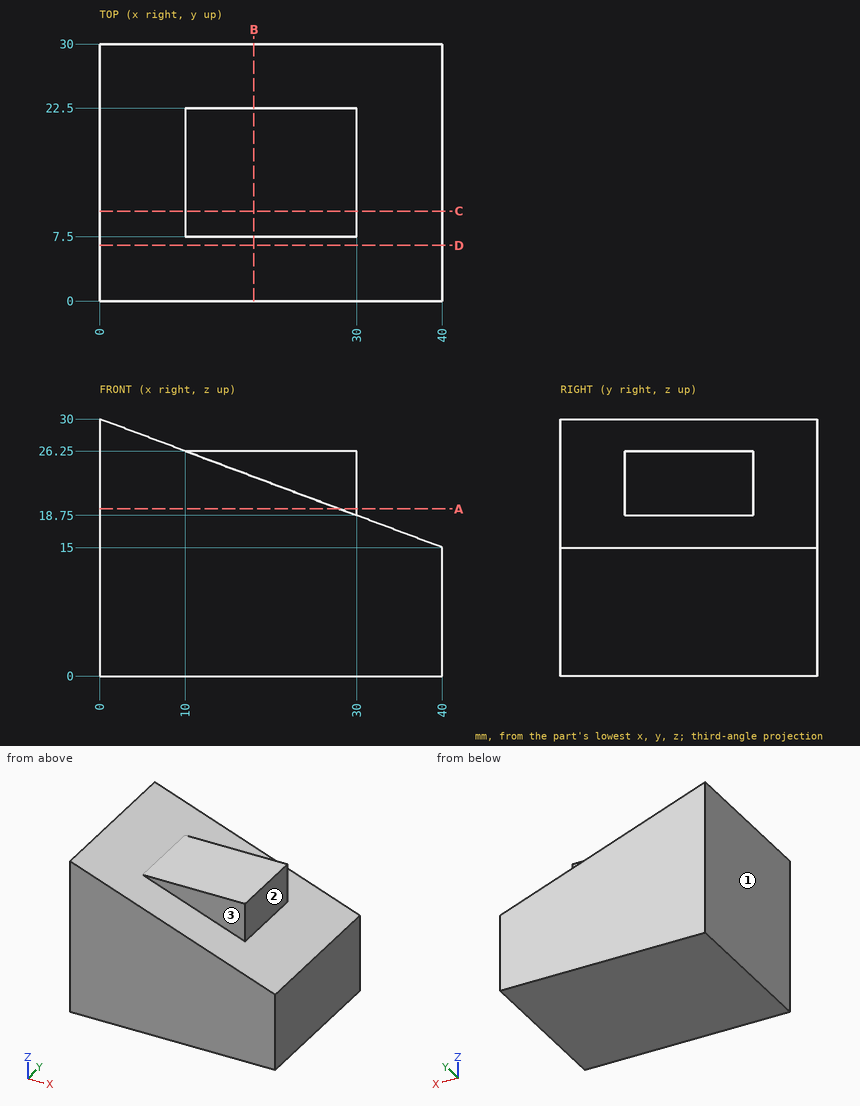
Here's the drawing with two shaded views (mm, measured from the low corner). I have some questions. A direction names the side the tool comes from. Coordinates: 2 decimals unless noted, no trailing zeros. Loops run counter-clockwise (first coordinate to the right, second up) from the corner with the lowest first, then second, coordinate; pieces in that order, holes last. Notation, with made-up numbers: M 71,-5.5 L 87,-5.5 A32 cw 87,30.5 Z; hole C -27,17 d3. An arc over 180 degrees is marked long. Return JSON: item names as keys, results as strings. Group by question number.
Item 1: Imagine slicing it at B-B (x = 18). Please give me the cut outline in (y, z), and give its area (4 significant figures).
Item 2: Imagine slicing it at A-A (z = 19.5). Please give me the cut outline in (x, y), and give its area (3 significant figures).
Item 3: Imagine slicing it at D-D (y = 6.5). Please give me the cut outline in (x, z).
Item 4: On a 3-axis mill with a long thin cutter (end or side, diameter ignored), from which of +Z, -Z, +X, -X, +Y, -Y can I reach the whole of each face in a straight line? I mean the marked faces 1, 2 and 3. Say none if no direction works.
Item 5: Imagine slicing it at C-C (y = 10.5). Please give me the cut outline in (x, z).
Item 6: If I drill on L1, parallel to Z at x = 23, y = 9.5; L2, parallel to X at y = 13.75, z = 20; L3, parallel to Z at x = 6, y = 4.5, over which ranges is the centre line in solid material (lowest first)? Write a range as from..to.
Item 7: I'm going to push flat-ended pins straight in: pin 1 Ø7.5 at (x, y) = (20, 13.5) entering from +Z; pin 2 Ø12 at (x, z) = (33.5, 24.5) entering from +Y; pin 3 Ø4 at (y, z) = (14.5, 22.5) entering from +X. Where does each tip first touch, or does it pass through?
Verdict:
{
 "1": {"outline": "M 0,0 L 30,0 L 30,23.25 L 22.5,23.25 L 22.5,26.25 L 7.5,26.25 L 7.5,23.25 L 0,23.25 Z", "area": "742.5 mm^2"},
 "2": {"outline": "M 0,0 L 28,0 L 28,7.5 L 30,7.5 L 30,22.5 L 28,22.5 L 28,30 L 0,30 Z", "area": "870 mm^2"},
 "3": {"outline": "M 0,0 L 40,0 L 40,15 L 0,30 Z"},
 "4": {"face 1": "+Z, -Z, -X, +Y, -Y", "face 2": "+Z, +X, +Y, -Y", "face 3": "+Z, +X, -Y"},
 "5": {"outline": "M 0,0 L 40,0 L 40,15 L 30,18.75 L 30,26.25 L 10,26.25 L 0,30 Z"},
 "6": {"L1": "z = 0..26.25", "L2": "x = 0..30", "L3": "z = 0..27.75"},
 "7": {"pin 1": "stops at z = 26.25", "pin 2": "stops at y = 22.5", "pin 3": "stops at x = 30"}
}
